```python
from build123d import *

# Parameters (mm, degrees)
SKETCH1_R           = 1
SKETCH1_R_2         = 0.3
BOSS_EXTRUDE1_DEPTH = 30.6
SKETCH2_W           = 20
SKETCH2_H           = 5.05
CUT_EXTRUDE1_DEPTH  = 0.5
SKETCH4_W           = 4.5
SKETCH4_H           = 0.5
CUT_EXTRUDE2_DEPTH  = 21.5
SKETCH5_R           = 1.7
CUT_EXTRUDE3_DEPTH  = 3
FILLET1_R           = 0.4
FILLET2_R           = 0.4


with BuildPart() as part:
    # Sketch1 → Boss-Extrude1 (new body)
    with BuildSketch(Plane.XY):
        with BuildLine():
            Line((-4.5, 2.25), (-4.5, 2.75))
            Line((-4.5, 2.75), (4.5, 2.75))
            Line((4.5, 2.75), (4.5, 2.25))
            ThreePointArc((4.5, 2.25), (5.207106781, 1.957106781), (5.5, 1.25))
            ThreePointArc((5.5, 1.25), (5.207106781, 0.542893219), (4.5, 0.25))
            Line((4.5, 0.25), (4.5, -0.75))
            Line((4.5, -0.75), (10, -0.75))
            Line((10, -0.75), (10, 7.25))
            Line((10, 7.25), (-10, 7.25))
            Line((-10, 7.25), (-10, -0.75))
            Line((-10, -0.75), (-4.5, -0.75))
            Line((-4.5, -0.75), (-4.5, 0.25))
            ThreePointArc((-4.5, 0.25), (-5.5, 1.25), (-4.5, 2.25))
        make_face()
        with BuildLine():
            Line((-4.5, 1.25), (-4.5, 2.25))
            ThreePointArc((-4.5, 2.25), (-5.5, 1.25), (-4.5, 0.25))
            Line((-4.5, 0.25), (-4.5, 1.25))
        make_face()
        with BuildLine():
            ThreePointArc((-3.545, 1.546605799), (-3.906959444, 2.05517259), (-4.5, 2.25))
            Line((-4.5, 2.25), (-4.5, 1.25))
            Line((-4.5, 1.25), (-4.5, 0.25))
            ThreePointArc((-4.5, 0.25), (-3.906959444, 0.44482741), (-3.545, 0.953394201))
            ThreePointArc((-3.545, 0.953394201), (-3.8, 1.25), (-3.545, 1.546605799))
        make_face()
        with Locations((-4.5, 1.25)):
            Circle(SKETCH1_R)
        with Locations((-3.5, 1.25)):
            Circle(SKETCH1_R_2)
        with Locations((3.5, 1.25)):
            Circle(SKETCH1_R_2)
        with Locations((4.5, 1.25)):
            Circle(SKETCH1_R)
        with BuildLine():
            Line((4.5, 0.25), (4.5, 2.25))
            ThreePointArc((4.5, 2.25), (3.906959444, 2.05517259), (3.545, 1.546605799))
            ThreePointArc((3.545, 1.546605799), (3.727486263, 1.445576072), (3.8, 1.25))
            ThreePointArc((3.8, 1.25), (3.727486263, 1.054423928), (3.545, 0.953394201))
            ThreePointArc((3.545, 0.953394201), (3.906959444, 0.44482741), (4.5, 0.25))
        make_face()
        with BuildLine():
            ThreePointArc((5.5, 1.25), (5.207106781, 1.957106781), (4.5, 2.25))
            Line((4.5, 2.25), (4.5, 0.25))
            ThreePointArc((4.5, 0.25), (5.207106781, 0.542893219), (5.5, 1.25))
        make_face()
    extrude(amount=BOSS_EXTRUDE1_DEPTH)

    # Sketch2 → Cut-Extrude1 (cut)
    with BuildSketch(Plane(origin=(0, 7.25, 0), x_dir=(1, 0, 0), z_dir=(0, 1, 0))):
        with Locations((0, -2.525)):
            Rectangle(SKETCH2_W, SKETCH2_H)
        with Locations((0, -28.075)):
            Rectangle(SKETCH2_W, SKETCH2_H)
    extrude(amount=-CUT_EXTRUDE1_DEPTH, mode=Mode.SUBTRACT)

    # Sketch4 → Cut-Extrude2 (cut)
    with BuildSketch(Plane.XY.offset(25.55)):
        with Locations((-2.25, 7)):
            Rectangle(SKETCH4_W, SKETCH4_H)
        with Locations((2.25, 7)):
            Rectangle(SKETCH4_W, SKETCH4_H)
    extrude(amount=-CUT_EXTRUDE2_DEPTH, mode=Mode.SUBTRACT)

    # Sketch5 → Cut-Extrude3 (cut)
    with BuildSketch(Plane(origin=(0, 7.25, 0), x_dir=(1, 0, 0), z_dir=(0, 1, 0))):
        with BuildLine():
            ThreePointArc((-7.5, -18.586900159), (-8.702081528, -21.488981687), (-5.8, -20.286900159))
            Line((-5.8, -20.286900159), (-7.5, -20.286900159))
            Line((-7.5, -20.286900159), (-7.5, -18.586900159))
        make_face()
        with BuildLine():
            Line((-7.5, -20.286900159), (-5.8, -20.286900159))
            ThreePointArc((-5.8, -20.286900159), (-6.297918472, -19.084818631), (-7.5, -18.586900159))
            Line((-7.5, -18.586900159), (-7.5, -20.286900159))
        make_face()
        with BuildLine():
            ThreePointArc((7.5, -18.586900159), (6.297918472, -19.084818631), (5.8, -20.286900159))
            Line((5.8, -20.286900159), (7.5, -20.286900159))
            Line((7.5, -20.286900159), (7.5, -18.586900159))
        make_face()
        with BuildLine():
            Line((7.5, -20.286900159), (5.8, -20.286900159))
            ThreePointArc((5.8, -20.286900159), (7.5, -21.986900159), (9.2, -20.286900159))
            ThreePointArc((9.2, -20.286900159), (8.702081528, -19.084818631), (7.5, -18.586900159))
            Line((7.5, -18.586900159), (7.5, -20.286900159))
        make_face()
        with BuildLine():
            ThreePointArc((9.2, -10.286900159), (7.5, -8.586900159), (5.8, -10.286900159))
            Line((5.8, -10.286900159), (7.5, -10.286900159))
            Line((7.5, -10.286900159), (7.5, -11.986900159))
            ThreePointArc((7.5, -11.986900159), (8.702081528, -11.488981687), (9.2, -10.286900159))
        make_face()
        with BuildLine():
            Line((7.5, -10.286900159), (5.8, -10.286900159))
            ThreePointArc((5.8, -10.286900159), (6.297918472, -11.488981687), (7.5, -11.986900159))
            Line((7.5, -11.986900159), (7.5, -10.286900159))
        make_face()
        with Locations(Location((-7.5, -10.286900159, 0), (0, 0, 90))):
            Circle(SKETCH5_R)
    extrude(amount=-CUT_EXTRUDE3_DEPTH, mode=Mode.SUBTRACT)

    # Fillet1
    fillet1_edges = [part.edges().sort_by_distance(p)[0] for p in [
        (-4.5, -0.75, 15.3),
        (-10, -0.75, 15.3),
        (10, -0.75, 15.3),
        (4.5, -0.75, 15.3),
        (-10, 7.25, 15.3),
        (10, 7.25, 15.3),
        (-10, 6.75, 2.525),
        (10, 6.75, 2.525),
        (10, 6.75, 28.075),
        (-10, 6.75, 28.075),
        (-4.5, 6.75, 15.3),
        (4.5, 7.25, 15.3),
    ]]
    fillet(fillet1_edges, radius=FILLET1_R)

    # Fillet2
    fillet2_edges = [part.edges().sort_by_distance(p)[0] for p in [
        (7.25, -0.75, 0),
        (7.25, -0.75, 30.6),
        (0, 6.75, 0),
        (10, 3, 0),
        (4.5, -0.05, 0),
        (-4.5, -0.05, 0),
        (-7.25, -0.75, 0),
        (-10, 3, 0),
        (-9.882842712, 6.632842712, 0),
        (9.882842712, 6.632842712, 0),
        (-9.882842712, -0.632842712, 0),
        (-4.617157288, -0.632842712, 0),
        (9.882842712, -0.632842712, 0),
        (4.617157288, -0.632842712, 0),
        (4.5, -0.05, 30.6),
        (10, 3, 30.6),
        (0, 6.75, 30.6),
        (-10, 3, 30.6),
        (-7.25, -0.75, 30.6),
        (-4.5, -0.05, 30.6),
        (-9.882842712, 6.632842712, 30.6),
        (9.882842712, 6.632842712, 30.6),
        (-9.882842712, -0.632842712, 30.6),
        (-4.617157288, -0.632842712, 30.6),
        (9.882842712, -0.632842712, 30.6),
        (4.617157288, -0.632842712, 30.6),
    ]]
    fillet(fillet2_edges, radius=FILLET2_R)


solid = part.part
```
For this review, take the finished solid that the model builds, in its own axes (mm). A direction names the side the tool comes from. Coordinates: 2 decimals unless noted, no trailing zeros. Order: outer loops, then holes, each group sorted by start corner. A loop starts at its lowest first (then second) coordinate and runs counter-clockwise, first axis right, second up. Notation, with made-up numbers: (7.25, 25) -> (62.25, 25) arc R33 ccw to (62.25, 56) -> close; hole circle Ø8 at (-11, -10). An arc over 180 degrees is marked (long way). Use CSV: the item, a comma, the result in double quotes. Start each with the question number.
Item 1: For faces 3 (the face through (-8, 4.25, 10)), 4 (the face through (-7, 7.25, 15)), 5 (the face through (0, 2.75, 15)), list the 3-axis set-ups (+Z, -Z, +X, -X, +Y, -Y) from which the entire face can be reached by the end or side of a thin tool; tool diameter is ignored.
Item 2: Wall thickness on probe 1 along Z at (x, y) = (-7.5, 6.15); probe 2 along X at (y, z) = (0, 23); probe 3 along Z at (x, y) = (-7.5, 6.55): over which ranges is each line inside the solid? List them lowest first.
Item 3: We need section C-C, the plane x = 1.25. Give the boundary of the cut face in (y, z).
Item 4: We need section B-B, the plane x = 4. Give the boundary of the cut face in (y, z), then the cut area to 3 significant figures.
Item 5: Insertion check: pin 1 (2.5 mm diameter, centred on x = 7.5, z = 10.5, fed in from +Y); pin 2 (2.5 mm diameter, centred on x = -1.5, z = 17, fed in from -Y); pin 3 (3 mm diameter, centred on x = -1, z = 7.5, fed in from +Y). Each pin has a flat end and moves straight along its axis. Give the tip position at first contact, or say it passes through.
Item 6: We need section A-A, the plane y = 5.5. Give the boundary of the cut face in (x, z), then the cut area to 3 significant figures.
Item 7: Draft analysis for pull direction X (two halves, no side actions). For faces 1 (the face through (0, 6.75, 15)), 2 (the face through (7, -0.75, 15)), state which applies: pulls with the +X half, pulls with the -X half, needs draft (parallel to the pull), parting line crosses it, or undercut.
Derived:
1,face 3,"+Y"
1,face 4,"+Z, -Z, +X, -X, +Y"
1,face 5,"+Z, -Z"
2,probe 1,"z = 0 to 8.59, 11.99 to 18.59, 21.99 to 30.6"
2,probe 2,"x = -10 to -4.5, 4.5 to 10"
2,probe 3,"z = 0.05 to 8.59, 11.99 to 18.59, 21.99 to 30.55"
3,outline,"(2.75, 0) -> (6.35, 0) arc R0.4 ccw to (6.75, 0.4) -> (6.75, 30.2) arc R0.4 ccw to (6.35, 30.6) -> (2.75, 30.6) -> close"
4,outline,"(0.38, 0) -> (2.12, 0) -> (2.12, 30.6) -> (0.38, 30.6) -> close; (2.75, 0) -> (6.35, 0) arc R0.4 ccw to (6.75, 0.4) -> (6.75, 30.2) arc R0.4 ccw to (6.35, 30.6) -> (2.75, 30.6) -> close"
4,area,"175 mm^2"
5,pin 1,"stops at y = 4.25"
5,pin 2,"stops at y = 2.75"
5,pin 3,"stops at y = 6.75"
6,outline,"(-10, 0.4) arc R0.4 ccw to (-9.6, 0) -> (9.6, 0) arc R0.4 ccw to (10, 0.4) -> (10, 30.2) arc R0.4 ccw to (9.6, 30.6) -> (-9.6, 30.6) arc R0.4 ccw to (-10, 30.2) -> close; hole circle Ø3.4 at (-7.5, 10.29); hole circle Ø3.4 at (-7.5, 20.29); hole circle Ø3.4 at (7.5, 10.29); hole circle Ø3.4 at (7.5, 20.29)"
6,area,"576 mm^2"
7,face 1,"undercut"
7,face 2,"needs draft"
